```python
from build123d import *

# Parameters (mm, degrees)
BASE_EXTRUDE_THIN_DEPTH = 31.75
CUT_EXTRUDE1_REACH      = 123.615
SKETCH2_R               = 6.35
BOSS_EXTRUDE1_DEPTH     = 3.175


with BuildPart() as part:
    # Sketch1 → Base-Extrude-Thin (new, symmetric)
    with BuildSketch(Plane(origin=(0, 0, 0), x_dir=(0, 0, -1), z_dir=(1, 0, 0))):
        with BuildLine():
            Line((-67.523772904, 7.427557692), (-25.673556457, 0.048235384))
            ThreePointArc((-25.673556457, 0.048235384), (-25.398942977, 0.012081834), (-25.122223493, 0))
            Line((-25.122223493, 0), (-3.175, 0))
            ThreePointArc((-3.175, 0), (-0.92993597, 0.92993597), (0, 3.175))
            Line((0, 3.175), (0, 79.375))
            ThreePointArc((0, 79.375), (-0.92993597, 81.62006403), (-3.175, 82.55))
            Line((-3.175, 82.55), (-57.15, 82.55))
            Line((-57.15, 82.55), (-57.15, 88.9))
            Line((-57.15, 88.9), (-3.175, 88.9))
            ThreePointArc((-3.175, 88.9), (3.560192091, 86.110192091), (6.35, 79.375))
            Line((6.35, 79.375), (6.35, 3.175))
            ThreePointArc((6.35, 3.175), (3.560192091, -3.560192091), (-3.175, -6.35))
            Line((-3.175, -6.35), (-25.122223493, -6.35))
            ThreePointArc((-25.122223493, -6.35), (-25.952381943, -6.313754499), (-26.776222386, -6.205293847))
            Line((-26.776222386, -6.205293847), (-68.626438832, 1.174028461))
            Line((-68.626438832, 1.174028461), (-67.523772904, 7.427557692))
        make_face()
    extrude(amount=BASE_EXTRUDE_THIN_DEPTH, both=True)

    # Sketch2 → Cut-Extrude1 (cut, up to next)
    with BuildSketch(Plane(origin=(0, 88.9, 0), x_dir=(-1, 0, 0), z_dir=(0, 1, 0)), mode=Mode.PRIVATE) as cut_extrude1_sk1:
        with Locations(Location((0, 38.1, 0), (0, 0, 90))):
            Circle(SKETCH2_R)
    cut_extrude1_tool1 = extrude(cut_extrude1_sk1.sketch, amount=-CUT_EXTRUDE1_REACH, mode=Mode.PRIVATE) & part.part
    add(cut_extrude1_tool1.solids().sort_by_distance((0, 88.9, 38.1))[0], mode=Mode.SUBTRACT)

    # Sketch3 → Boss-Extrude1 (add)
    with BuildSketch(Plane(origin=(31.75, 0, 0), x_dir=(0, 0, -1), z_dir=(1, 0, 0))):
        with BuildLine():
            Line((-19.05, 0), (-3.175, 0))
            ThreePointArc((-3.175, 0), (-0.92993597, 0.92993597), (0, 3.175))
            Line((0, 3.175), (0, 25.4))
            Line((0, 25.4), (-19.05, 0))
        make_face()
    boss_extrude1 = extrude(amount=-BOSS_EXTRUDE1_DEPTH)

    # Mirror1: Boss-Extrude1 across plane
    add(boss_extrude1.mirror(Plane(origin=(0, 0, 0), x_dir=(0, 0, 1), z_dir=(1, 0, 0))))


solid = part.part
```
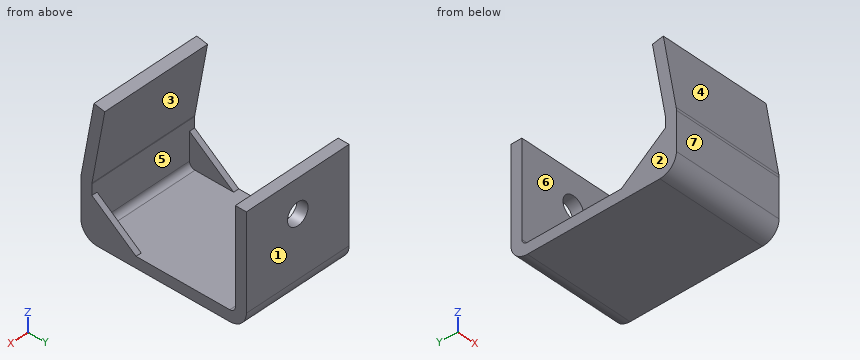
Part model, mm, in its own coordinate system. Face numbers are marked on the shaded views. A direction names the side the tool comes from. Round coordinates to 2 decimals unless told otherwise and drop trailing zeros. Write each loop counter-clockwise with the first axis right and the second up, starting at its lowest first coordinate (ties: lowest second). Pieces come first, ordered by that corner, then holes. Notation, with made-up numbers: M -37.75,58.25 L 11.25,58.25 A9 cw 11.25,68.25 Z; hole C 89.25,81.5 d1. An arc over 180 degrees is marked long. Answer as CSV lines item,"result". Start each with the question number.
1) Band-saw the part on C-C (z = 38.1). List the corners of the cut face in (x, y), then the cut area to 3 significant figures.
2) Which spindle directions (+Z, -Z, +X, -X, +Y, -Y) get a long thin tool onto all of the face, cutting with end or side? Do the marked faces 5, 6 and 7. Say none if no direction does.
3) Band-saw the part on B-B (z = 6). List the corners of the cut face in (x, y) (3 decimals), then the cut area to 3 significant figures.
4) Band-saw the part on D-D (x = -24.5). List the corners of the cut face in (y, z) (3 decimals), then the cut area to 3 significant figures.
5) Drop flat-ended pins along their axis: pin 1 (10 mm diameter, centred on x = 0, z = 38.1, fed in from -Y); pin 2 (3 mm diameter, centred on x = -14, y = 49.5, fed in from +Z); pin 3 (7 mm diameter, centred on x = 9.5, y = 86, fed in from +Z). Give the stop position or say it passes through.
6) Mould opens along Y. For the marked faces 1, 2, 3 and 4 say: +Y half, -Y half, draft (parallel to the pull), parting line (faces both ways), or undercut.
7) Band-saw the part on A-A (x = 0). List the corners of the cut face in (y, z) (3 decimals).
8) Drill centre lines: L1, parallel to Y at x = 13, z = 20; L2, parallel to X at y = 84.75, z = 38.1; L3, parallel to Z at x = 8.5, y = 78. Where is each one in solid material? Low to high.
Worked out:
1,outline,"M -31.75,-4.21 L 31.75,-4.21 L 31.75,2.24 L -31.75,2.24 Z; M -31.75,82.55 L -6.35,82.55 L -6.35,88.9 L -31.75,88.9 Z; M 6.35,82.55 L 31.75,82.55 L 31.75,88.9 L 6.35,88.9 Z"
1,area,"732 mm²"
2,face 5,"none"
2,face 6,"+Z, +X, -X"
2,face 7,"+Z, -Z, +X, -X, -Y"
3,outline,"M -31.75,-6.35 L 31.75,-6.35 L 31.75,17.4 L 28.575,17.4 L 28.575,0 L -28.575,0 L -28.575,17.4 L -31.75,17.4 Z; M -31.75,82.55 L 31.75,82.55 L 31.75,88.9 L -31.75,88.9 Z"
3,area,"917 mm²"
4,outline,"M -6.35,3.175 A9.525 ccw 3.175,-6.35 L 79.375,-6.35 A9.525 ccw 88.9,3.175 L 88.9,57.15 L 82.55,57.15 L 82.55,3.175 A3.175 cw 79.375,0 L 3.175,0 A3.175 cw 0,3.175 L 0,25.122 A3.175 cw 0.048,25.674 L 7.428,67.524 L 1.174,68.626 L -6.205,26.776 A9.525 ccw -6.35,25.122 Z"
4,area,"1,370 mm²"
5,pin 1,"y = -5.09"
5,pin 2,"z = 0"
5,pin 3,"z = 57.15"
6,face 1,"+Y half"
6,face 2,"draft"
6,face 3,"undercut"
6,face 4,"-Y half"
7,outline,"M -6.35,3.175 A9.525 ccw 3.175,-6.35 L 79.375,-6.35 A9.525 ccw 88.9,3.175 L 88.9,31.75 L 82.55,31.75 L 82.55,3.175 A3.175 cw 79.375,0 L 3.175,0 A3.175 cw 0,3.175 L 0,25.122 A3.175 cw 0.048,25.674 L 7.428,67.524 L 1.174,68.626 L -6.205,26.776 A9.525 ccw -6.35,25.122 Z; M 82.55,44.45 L 88.9,44.45 L 88.9,57.15 L 82.55,57.15 Z"
8,L1,"-6.35 to 0, 82.55 to 88.9"
8,L2,"-31.75 to -6.35, 6.35 to 31.75"
8,L3,"-6.35 to 0"
